Build history of the part. All positions in model axes, mm. Face numbers are marked on the shaded views. A direction names the side the tool comes from. Give positions to 0.01 mm unless a question says otherwise; leave off trailing zeros. Order: outer loops, then holes, each group sorted by start corner. A loop starts at its lowest first (then second) coordinate and runs counter-clockwise, first axis right, second up. Notation, with made-up numbers: (17.5, -33.75) - (39.5, -33.75) arc R11 ccw to (39.5, -13.75) - close; hole circle Ø11 at (0, 48). An arc over 180 degrees is marked (long way). Use a Markdown table: item, result. Add a question column.
(1) Wall check: line 1 (X direction, y = 29.6, z = 0); line 2 (Z direction, x = 0, y = 8.25). Give the ranges that are in metal, low to high.
(2) Slice it at D-D (y = 27). Write the cut outline in (x, z), then the cut area to 3 significant figures.
(3) Slice it at C-C (y = 3.5). Write the cut outline in (x, z), then the cut area to 3 significant figures.
(4) Mould opens along Z. For the marked faces 1, 2 and 3 say: +Z half, -Z half, draft (parallel to the pull), parting line (faces both ways), or undercut.
(5) Flat gauge pins, fed straight in: pin 1 (13 mm diameter, centred on x = 11.31, z = 11.31, fed in from +Y); pin 2 (12 mm diameter, centred on y = 22, z = -9.5, fed in from -X); pin 3 (6 mm diameter, centred on x = -11.31, z = 11.31, fed in from +Y); pin 4 (4 mm diameter, centred on x = -12, z = 13, fed in from -Y). Where does each tip first touch, or does it go through?
(6) Which spindle directions (+Z, -Z, +X, -X, +Y, -Y) get a long thin tool onto all of the face, cutting with end or side? Do the marked faces 4, 5 and 6. Say none if no direction does.
from build123d import *

# Parameters (mm, degrees)
FLANGE_START         = 6
FLANGE_DEPTH         = 6
SKETCH9_R            = 4
COUNTERBORE_DEPTH    = 4.1
SKETCH10_R           = 2.25
MOUNTING_HOLES_DEPTH = 35.392004885
SKETCH11_R           = 0.375
CHAMFER1_SIZE        = 0.2


with BuildPart() as part:
    # Sketch5 → Bearing Body (revolve)
    with BuildSketch(Plane(origin=(0, 0, 0), x_dir=(0, 0, -1), z_dir=(1, 0, 0))):
        Polygon((6.5, 30), (6, 30), (6, 0), (6.5, 0), (6.5, 0.8), (10, 0.8), (10, 0), (10.5, 0), (10.5, 30), (10, 30), (10, 29.2), (6.5, 29.2), align=None)
    revolve(axis=Axis((0, 0, 0), (0, 1, 0)))

    # Sketch8 → Flange (add)
    with BuildSketch(Plane(origin=(0, 0, 0), x_dir=(1, 0, 0), z_dir=(0, 1, 0)).offset(FLANGE_START)):
        Polygon((0, -16), (-14, -16), (-16, -14), (-16, 0), (-16, 14), (-14, 16), (0, 16), (14, 16), (16, 14), (16, 0), (16, -14), (14, -16), align=None)
        with BuildLine():
            ThreePointArc((-10.5, 0), (-7.424621202, -7.424621202), (0, -10.5))
            ThreePointArc((0, -10.5), (7.424621202, -7.424621202), (10.5, 0))
            ThreePointArc((10.5, 0), (7.424621202, 7.424621202), (0, 10.5))
            ThreePointArc((0, 10.5), (-7.424621202, 7.424621202), (-10.5, 0))
        make_face(mode=Mode.SUBTRACT)
    extrude(amount=-FLANGE_DEPTH)

    # Sketch9 → Counterbore (cut)
    with BuildSketch(Plane(origin=(0, 0, 0), x_dir=(-1, 0, 0), z_dir=(0, -1, 0))):
        with Locations(Location((11.313708499, -11.313708499, 0), (0, 0, 90))):
            Circle(SKETCH9_R)
        with Locations(Location((-11.313708499, -11.313708499, 0), (0, 0, 90))):
            Circle(SKETCH9_R)
        with Locations(Location((-11.313708499, 11.313708499, 0), (0, 0, 90))):
            Circle(SKETCH9_R)
        with Locations(Location((11.313708499, 11.313708499, 0), (0, 0, 90))):
            Circle(SKETCH9_R)
    extrude(amount=-COUNTERBORE_DEPTH, mode=Mode.SUBTRACT)

    # Sketch10 → Mounting Holes (cut, through all)
    with BuildSketch(Plane(origin=(0, 4.1, 0), x_dir=(-1, 0, 0), z_dir=(0, -1, 0))):
        with Locations(Location((11.313708499, 11.313708499, 0), (0, 0, 90))):
            Circle(SKETCH10_R)
        with Locations(Location((11.313708499, -11.313708499, 0), (0, 0, 90))):
            Circle(SKETCH10_R)
        with Locations(Location((-11.313708499, -11.313708499, 0), (0, 0, 90))):
            Circle(SKETCH10_R)
        with Locations(Location((-11.313708499, 11.313708499, 0), (0, 0, 90))):
            Circle(SKETCH10_R)
    extrude(amount=-MOUNTING_HOLES_DEPTH, mode=Mode.SUBTRACT)

    # Sketch11 → Relief (revolve, cut)
    with BuildSketch(Plane(origin=(0, 0, 0), x_dir=(0, 0, -1), z_dir=(1, 0, 0)), mode=Mode.PRIVATE) as relief_sk:
        with Locations((-10.5, 6)):
            Circle(SKETCH11_R)
    revolve(relief_sk.sketch.rotate(Axis((0, 0, 0), (0, 1, 0)), 180), axis=Axis((0, 0, 0), (0, 1, 0)), mode=Mode.SUBTRACT)

    # Chamfer1
    chamfer1_edges = [part.edges().sort_by_distance(p)[0] for p in [
        (-15, 6, 15),
        (0, 6, 16),
        (15, 6, 15),
        (16, 6, 0),
        (15, 6, -15),
        (0, 6, -16),
        (-15, 6, -15),
        (-16, 6, 0),
        (-15, 0, 15),
        (0, 0, 16),
        (15, 0, 15),
        (16, 0, 0),
        (15, 0, -15),
        (0, 0, -16),
        (-15, 0, -15),
        (-16, 0, 0),
    ]]
    chamfer(chamfer1_edges, length=CHAMFER1_SIZE)


solid = part.part
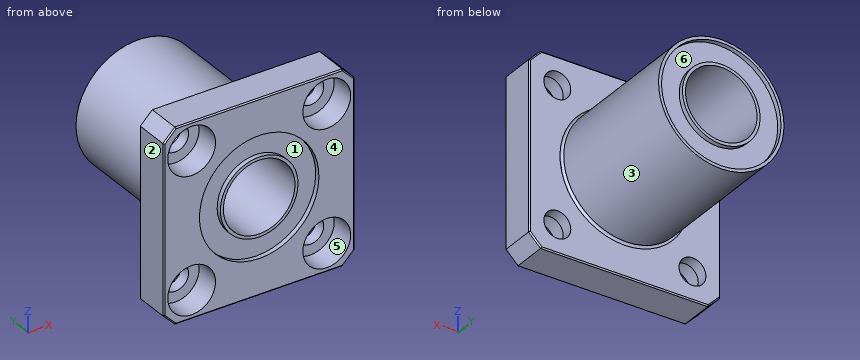
Solution:
| question | item | result |
|---|---|---|
| 1 | line 1 | -10.5 to -10, -6.5 to -6, 6 to 6.5, 10 to 10.5 |
| 1 | line 2 | -10.5 to -6, 6 to 10.5 |
| 2 | outline | circle Ø21 at (0, 0); hole circle Ø12 at (0, 0) |
| 2 | area | 233 mm2 |
| 3 | outline | (-16, -14) - (-14, -16) - (14, -16) - (16, -14) - (16, 14) - (14, 16) - (-14, 16) - (-16, 14) - close; hole circle Ø8 at (-11.31, -11.31); hole circle Ø8 at (-11.31, 11.31); hole circle Ø12 at (0, 0); hole circle Ø8 at (11.31, -11.31); hole circle Ø8 at (11.31, 11.31) |
| 3 | area | 702 mm2 |
| 4 | face 1 | undercut |
| 4 | face 2 | draft |
| 4 | face 3 | parting line |
| 5 | pin 1 | y = 30 |
| 5 | pin 2 | x = -9.9 |
| 5 | pin 3 | y = 6 |
| 5 | pin 4 | y = 4.1 |
| 6 | face 4 | +Z, -Z, +X, -X, -Y |
| 6 | face 5 | -Y |
| 6 | face 6 | +Y |
